Job drawing, mm, ordinate dimensions from the low corner. One solid piece. A direction names the side the tool comes from. Round coordinates to 2 decimals unless told otherwise and drop trailing zeros. Order: outer loops, then holes, each group sorted by start corner. A loop starts at its lowest first (then second) coordinate and runs counter-clockwise, first axis right, second up. Notation, with made-up numbers: (68.5, -34.5) -> (112.5, -34.5) arc R22 ccw to (112.5, -9.5) -> close; hole circle Ø6 at (-8, 81). An arc over 180 degrees is marked (long way). Return JSON: item names as keys, results as strings. Group by question number.
Q1. Cut at D-D (z = 44.5). Write the cut outline in (x, y) (1 decimal), then the cut area to 3 significant figures.
Q2. Mould opens along Z. For the marked faces 1, 2 and 3 say: +Z half, -Z half, draft (parallel to the pull), parting line (faces both ways), or undercut.
Q3. Probe line 1 along Z through (x, y) = (63, 9.5); line 2 along X through (y, z) = (20.5, 61.5) (1 decimal); line 3 along Z through (x, y) = (41, 14.75) (1 decimal). List the from-to ranges inside material, lowest first.
Q4. Cut at B-B (y = 19.25). Write the cut outline in (x, z), then the cut area to 3 significant figures.
Q5. Cut at C-C (x = 101). Write the cut outline in (y, z) (1 decimal).
Q6. Which spindle directions (+Z, -Z, +X, -X, +Y, -Y) get a long thin tool onto all of the face, cutting with end or side? Do the marked faces 4 and 5. Say none if no direction does.
Q7. Flat gauge pins, fed straight in: pin 1 (6 mm diameter, centred on y = 19, z = 67.5, fed in from -X); pin 2 (2 mm diameter, centred on y = 20, z = 27.5, fed in from -X); pin 3 (8 mm diameter, centred on x = 53, y = 12, fed in from -Z). Where does each tip first touch, or does it go through?
Q8. Cut at A-A (z = 71). Write the cut outline in (x, y) (1 decimal).
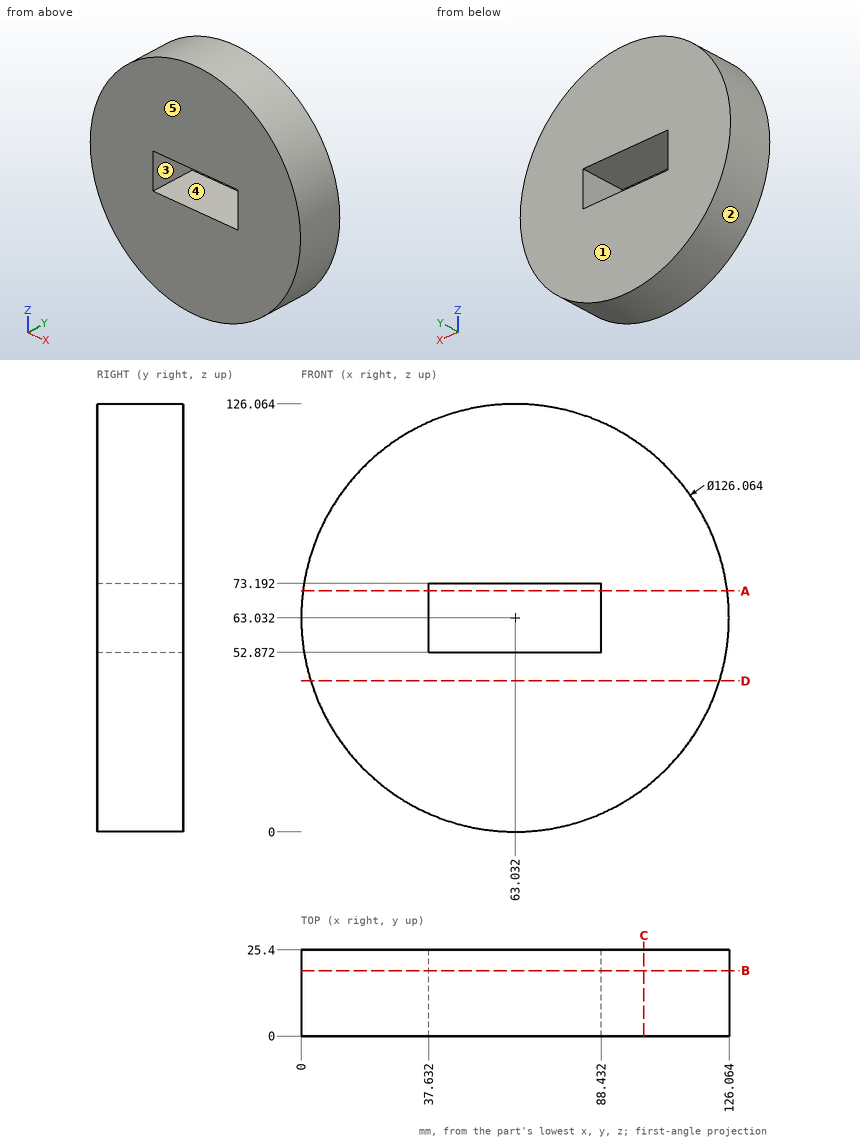
Solution:
{
 "1": {"outline": "(2.8, 0) -> (123.3, 0) -> (123.3, 25.4) -> (2.8, 25.4) -> close", "area": "3,060 mm²"},
 "2": {"face 1": "draft", "face 2": "parting line", "face 3": "undercut"},
 "3": {"line 1": "z = 0 to 52.87, 73.19 to 126.06", "line 2": "x = 0 to 37.6, 88.4 to 126", "line 3": "z = 4 to 52.9, 73.2 to 122.1"},
 "4": {"outline": "circle Ø126.06 at (63.03, 63.03); hole (37.63, 52.87) -> (88.43, 52.87) -> (88.43, 73.19) -> (37.63, 73.19) -> close", "area": "11,400 mm²"},
 "5": {"outline": "(0, 12.7) -> (25.4, 12.7) -> (25.4, 113.3) -> (0, 113.3) -> close"},
 "6": {"face 4": "+Y, -Y", "face 5": "+Z, -Z, +X, -X, -Y"},
 "7": {"pin 1": "stops at x = 0.02", "pin 2": "stops at x = 10.3", "pin 3": "stops at z = 0.29"},
 "8": {"outline": "(0.5, 0) -> (37.6, 0) -> (37.6, 25.4) -> (0.5, 25.4) -> close; (88.4, 0) -> (125.6, 0) -> (125.6, 25.4) -> (88.4, 25.4) -> close"}
}
